Verification items for the finished model (mm, model axes). A direction names the side the tool comes from. Give positions to 0.01 mm unless a question says otherwise; leave off trailing zeros. Loops run counter-clockwise (first coordinate to the right, second up) from the corner with the lowest first, then second, coordinate; pieces in that order, holes last. Notation, with made-up numbers: M 63.5,25.5 L 70.5,25.5 A21 ccw 70.5,31.5 Z; hole C 47,8 d2. An arc over 180 degrees is marked long. Use CSV: the item, a comma, the result in double quotes.
from build123d import *

# Parameters (mm, degrees)
BOSS_EXTRUDE2_DEPTH = 1.65
BOSS_EXTRUDE3_DEPTH = 7
BOSS_EXTRUDE4_DEPTH = 3.2
SKETCH7_W           = 40
SKETCH7_H           = 2.5
BOSS_EXTRUDE5_DEPTH = 4
SKETCH8_W           = 40
SKETCH8_H           = 19.15
BOSS_EXTRUDE6_DEPTH = 11.1
SKETCH9_W           = 4.8
SKETCH9_H           = 2.5
BOSS_EXTRUDE7_DEPTH = 6


with BuildPart() as part:
    # Sketch3 → Boss-Extrude2 (new body)
    with BuildSketch(Plane(origin=(0, 0, 0), x_dir=(1, 0, 0), z_dir=(0, 1, 0))):
        Polygon((0, 0), (0, 36.15), (80, 36.15), (80, 20.120748629), (80, 16.120748629), (80, 0), align=None)
    extrude(amount=-BOSS_EXTRUDE2_DEPTH)

    # Sketch5 → Boss-Extrude3 (add)
    with BuildSketch(Plane(origin=(0, 0, 0), x_dir=(1, 0, 0), z_dir=(0, 1, 0))):
        Polygon((75.75, 11.070748629), (75.75, 5.925), (4.25, 5.925), (4.25, 30.225), (75.75, 30.225), (75.75, 25.170748629), align=None)
    extrude(amount=BOSS_EXTRUDE3_DEPTH)

    # Sketch6 → Boss-Extrude4 (add)
    with BuildSketch(Plane(origin=(0, 0, 0), x_dir=(1, 0, 0), z_dir=(0, 1, 0))):
        Polygon((80, 20.120748629), (80, 16.120748629), (75.75, 11.070748629), (75.75, 25.170748629), align=None)
    extrude(amount=BOSS_EXTRUDE4_DEPTH)

    # Sketch7 → Boss-Extrude5 (add)
    with BuildSketch(Plane(origin=(0, 0, 0), x_dir=(1, 0, 0), z_dir=(0, 1, 0))):
        with Locations((27.25, 34.9)):
            Rectangle(SKETCH7_W, SKETCH7_H)
    extrude(amount=BOSS_EXTRUDE5_DEPTH)

    # Sketch8 → Boss-Extrude6 (add)
    with BuildSketch(Plane.XZ.offset(1.65)):
        with Locations((27.25, -26.575)):
            Rectangle(SKETCH8_W, SKETCH8_H)
    extrude(amount=BOSS_EXTRUDE6_DEPTH)

    # Sketch9 → Boss-Extrude7 (add)
    with BuildSketch(Plane(origin=(47.25, 0, 0), x_dir=(0, 0, -1), z_dir=(1, 0, 0))):
        with Locations((26.575, -11.5)):
            Rectangle(SKETCH9_W, SKETCH9_H)
    extrude(amount=BOSS_EXTRUDE7_DEPTH)


solid = part.part
(1) Section check C-C on z = -10. Record the cut outline in (x, y).
Calculated:
outline,"M 0,-1.65 L 80,-1.65 L 80,0 L 75.75,0 L 75.75,7 L 4.25,7 L 4.25,0 L 0,0 Z"
(2) Mould release check, pull along Z, two halves, no side actions. Record for faces 1 (the flat face through (39, 3, -30.225)), 2 (the flat face through (47.25, -7, -27)), 3 (the flat face through (27, -7, -17)): released by +Z, released by -Z, zero draft, split by the parting line, or undercut.
Calculated:
face 1,"undercut"
face 2,"zero draft"
face 3,"released by +Z"
(3) Section check D-D on y = -6.5. Record the cut outline in (x, z).
Calculated:
outline,"M 7.25,-36.15 L 47.25,-36.15 L 47.25,-17 L 7.25,-17 Z"
(4) Section check B-B on x = 23. Record the cut outline in (y, z) (3 decimals), plus the area to 3 significant figures.
Calculated:
outline,"M -12.75,-36.15 L 4,-36.15 L 4,-33.65 L 0,-33.65 L 0,-30.225 L 7,-30.225 L 7,-5.925 L 0,-5.925 L 0,0 L -1.65,0 L -1.65,-17 L -12.75,-17 Z"
area,"452 mm²"
(5) Section check A-A on y = 1.25. Record the cut outline in (x, z) (3 decimals).
Calculated:
outline,"M 4.25,-30.225 L 75.75,-30.225 L 75.75,-25.171 L 80,-20.121 L 80,-16.121 L 75.75,-11.071 L 75.75,-5.925 L 4.25,-5.925 Z; M 7.25,-36.15 L 47.25,-36.15 L 47.25,-33.65 L 7.25,-33.65 Z"
(6) Scan lines: L1, parallel to Z at x = 8, y = 1.5 (3 decimals); L2, parallel to X at y = -8.25, z = -32.5; L3, parallel to Y at x = 57, z = -20.5. Record each from-to range of solid material in increasing order. Write a range as from..to.
Calculated:
L1,"z = -36.15..-33.65, -30.225..-5.925"
L2,"x = 7.25..47.25"
L3,"y = -1.65..7"
(7) Tool access check on faces 4 (the flat face through (7.25, 2, -35)), 5 (the flat face through (7.25, -7, -27)), 6 (the flat face through (50, -12, -24.175)), 7 (the flat face through (77.905, 1.578, -13.631)). Record the directions out of +Z, -Z, +X, -X, +Y, -Y that give a thin tool (end or side, any length) a straight path to the whole face; none if there is none.
Calculated:
face 4,"-Z, -X, +Y"
face 5,"+Z, -Z, -X, -Y"
face 6,"+Z, +X, -Y"
face 7,"+Z, +X, +Y"
(8) Depth check by flat-ended pin: pin 1 Ø1 at (x, z) = (30, -14) entering from -Y; pin 2 Ø3 at (x, y) = (24, 2) entering from +Z (3 decimals); pin 3 Ø0.8 at (y, z) = (2, -35.5) entering from +X. Enter the tip coordinate at first touch or a pass-through.
Calculated:
pin 1,"stops at y = -1.65"
pin 2,"stops at z = -5.925"
pin 3,"stops at x = 47.25"
